from build123d import *

# Parameters (mm, degrees)
ESBO_O1_R                = 5.5
RESSALTO_EXTRUS_O1_DEPTH = 6
FILETE1_R                = 1.75


with BuildPart() as part:
    # Esboço1 → Ressalto-extrusão1 (new body)
    with BuildSketch(Plane(origin=(0, 0, 0), x_dir=(1, 0, 0), z_dir=(0, 1, 0))):
        Polygon((-13, -13), (13, -13), (13, -5.242288745), (10, -5.242288745), (10, -1.742288745), (13, -1.742288745), (13, 13), (-13, 13), (-13, -1.742288745), (-10, -1.742288745), (-10, -5.242288745), (-13, -5.242288745), align=None)
        with Locations(Location((0, -3.5, 0), (0, 0, 270))):
            Circle(ESBO_O1_R, mode=Mode.SUBTRACT)
        Polygon((-5.5, 10), (0, 10), (5.5, 10), (5.5, 4), (-5.5, 4), align=None, mode=Mode.SUBTRACT)
    extrude(amount=RESSALTO_EXTRUS_O1_DEPTH)

    # Filete1
    filete1_edges = [part.edges().sort_by_distance(p)[0] for p in [
        (10, 3, 1.742288745),
        (10, 3, 5.242288745),
        (-10, 3, 1.742288745),
        (-10, 3, 5.242288745),
    ]]
    fillet(filete1_edges, radius=FILETE1_R - 0.0001)  # a hair under: the kernel refuses the full size


solid = part.part
Work out the finished part from the listing and answer in its coordinate system (mm). A direction names the side the tool comes from. Round coordinates to 2 decimals unless told otherwise and drop trailing zeros. Write each loop counter-clockwise with the first axis right and the second up, starting at its lowest first coordinate (ties: lowest second). Pieces come first, ordered by that corner, then holes.
1) The mould has two halves that part along Z. Classify faces 4 (the flat face through (13, 3, -6)), 5 (the flat face through (-12, 3, 5.242)), 6 (the flat face through (0, 3, -13)): pulls with the +Z half, pulls with the -Z half, needs draft (parallel to the pull), parting line crosses it, or undercut.
2) Straight lines are drawn through the part: line 1 (X direction, y = 2.5, z = 3.5); line 2 (X direction, y = 5.3, z = -7.25); line 3 (Z direction, x = 4.5, y = 1.1). For each, find the intervals that lie inside material, in ascending order.
3) A cutting plane is placed at C-C (z = 3). Give the vertices of the cut face in (x, y).
4) A tool of negligible diameter and unlimited length cuts with its end or side. For faces 1 (the cylindrical face through (10.526, 3.042, 4.743)), 2 (the cylindrical face through (-10.53, 3.04, 2.24)), 3 (the flat face through (0, 3, -10)), from which of +Z, -Z, +X, -X, +Y, -Y can it reach the whole face along a straight path? Write none if from no direction.
5) A cutting plane is placed at B-B (x = 0). Give the vertices of the cut face in (y, z).
6) A cutting plane is placed at A-A (y = 3.35). Give the number of separate pieces and of enclosed holes in the cut face, plus the area to 3 significant figures.
7) A cutting plane is placed at D-D (x = 5). Give the vertices of the cut face in (y, z), plus the area to 3 significant figures.
Completed:
1. face 4: needs draft
1. face 5: undercut
1. face 6: pulls with the -Z half
2. line 1: x = -10 to -5.5, 5.5 to 10
2. line 2: x = -13 to -5.5, 5.5 to 13
2. line 3: z = -13 to -10, -4 to 0.34, 6.66 to 13
3. outline: (-10.07, 0) - (-5.48, 0) - (-5.48, 6) - (-10.07, 6) - close; (5.48, 0) - (10.07, 0) - (10.07, 6) - (5.48, 6) - close
4. face 1: +X, +Y, -Y
4. face 2: -X, +Y, -Y
4. face 3: +Y, -Y
5. outline: (0, -13) - (6, -13) - (6, -10) - (0, -10) - close; (0, -4) - (6, -4) - (6, -2) - (0, -2) - close; (0, 9) - (6, 9) - (6, 13) - (0, 13) - close
6. separate pieces: 1
6. enclosed holes: 2
6. area: 497 mm2
7. outline: (0, -13) - (6, -13) - (6, -10) - (0, -10) - close; (0, -4) - (6, -4) - (6, 1.21) - (0, 1.21) - close; (0, 5.79) - (6, 5.79) - (6, 13) - (0, 13) - close
7. area: 92.5 mm2
